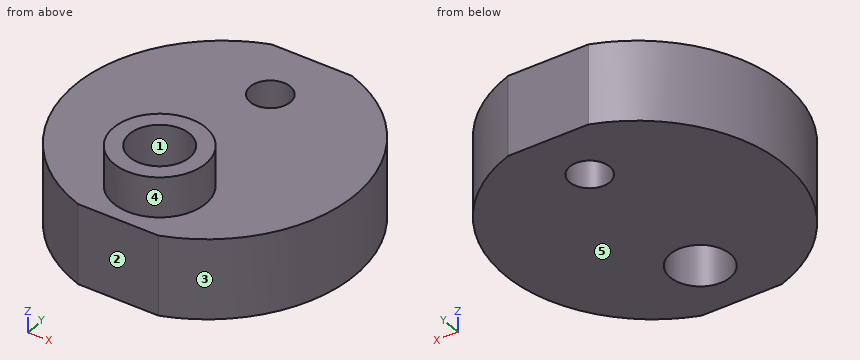
from build123d import *

# Parameters (mm, degrees)
MODEL_R             = 7.3025
MODEL_R_2           = 3.175
MODEL_R_3           = 4.7625
BOSS_EXTRUDE1_DEPTH = 12.7
MODEL_3_R           = 7.3025
MODEL_3_R_2         = 4.7625
BOSS_EXTRUDE2_DEPTH = 19.05


with BuildPart() as part:
    # Model → Boss-Extrude1 (new body)
    # profile 1 of 2: a face of its own
    with BuildSketch(Plane.XY):
        with BuildLine():
            Line((277.621999997, 256.159), (264.921999997, 256.159))
            ThreePointArc((264.921999997, 256.159), (249.046999977, 233.934), (264.921999997, 211.709))
            Line((264.921999997, 211.709), (277.621999997, 211.709))
            ThreePointArc((277.621999997, 211.709), (293.497000017, 233.934), (277.621999997, 256.159))
        make_face()
        with Locations((271.271999997, 221.234)):
            Circle(MODEL_R, mode=Mode.SUBTRACT)
        with Locations((271.271999997, 246.634)):
            Circle(MODEL_R_2, mode=Mode.SUBTRACT)
    # profile 2 of 2: a face of its own
    with BuildSketch(Plane.XY):
        with Locations((271.271999997, 221.234)):
            Circle(MODEL_R)
        with Locations((271.271999997, 221.234)):
            Circle(MODEL_R_3, mode=Mode.SUBTRACT)
    extrude(amount=BOSS_EXTRUDE1_DEPTH)

    # Model_3 → Boss-Extrude2 (add)
    with BuildSketch(Plane.XY):
        with Locations(Location((271.271999997, 221.234, 0), (0, 0, 180))):
            Circle(MODEL_3_R)
        with Locations((271.271999997, 221.234)):
            Circle(MODEL_3_R_2, mode=Mode.SUBTRACT)
    extrude(amount=BOSS_EXTRUDE2_DEPTH)


solid = part.part
For this review, take the finished solid that the model builds, in its own axes (mm). Face numbers are marked on the shaded views. A direction names the side the tool comes from. Round coordinates to 2 decimals unless told otherwise and drop trailing zeros. Write each loop counter-clockwise with the first axis right and the second up, starting at its lowest first coordinate (ties: lowest second). Pieces come first, ordered by that corner, then holes. Notation, with made-up numbers: (11.25, 35) -> (17.25, 35) arc R19 cw to (17.25, 69) -> close; hole circle Ø1 at (24.25, 45.5). An arc over 180 degrees is marked (long way). Put each result on its own line as item: value.
Q1. Consider section B-B on x = 272.5. State the section outline as (y, z) points.
Determined:
outline: (211.71, 0) -> (216.63, 0) -> (216.63, 19.05) -> (214.04, 19.05) -> (214.04, 12.7) -> (211.71, 12.7) -> close; (225.84, 0) -> (243.71, 0) -> (243.71, 12.7) -> (228.43, 12.7) -> (228.43, 19.05) -> (225.84, 19.05) -> close; (249.56, 0) -> (256.16, 0) -> (256.16, 12.7) -> (249.56, 12.7) -> close
Q2. To check wall thickness, follow L1, parallel to Y at x = 271, z = 5; L2, parallel to X at y = 221, z = 17.25; L3, parallel to Z at x = 269, y = 236.5. State the ranges of each line that lie inside material, in increasing order. Write a range as [from, to].
Determined:
L1: y = [211.71, 216.48], [225.99, 243.47], [249.8, 256.16]
L2: x = [263.97, 266.52], [276.03, 278.57]
L3: z = [0, 12.7]
Q3. Consider section C-C on z = 9. Give the number of separate pieces and of enclosed holes in the cut face, and give its area (3 significant figures).
Determined:
separate pieces: 1
enclosed holes: 2
area: 1,490 mm^2
Q4. Machinability: for the marked faces 4 and 5, which of the approach directions +Z, -Z, +X, -X, +Y, -Y give a long, thin tool a straight path to every point of the face, cutting with its end or side? Answer none if there is none.
Determined:
face 4: +Z
face 5: -Z, +X, -X, +Y, -Y
Q5. Clearance check with flat-ended pins moving along their axes: pin 1 Ø6 at (y, z) = (229, 3.5) entering from +X; pin 2 Ø8 at (x, y) = (286, 239) entering from +Z; pin 3 Ø4 at (y, z) = (220, 8) entering from -X. State where each tip first meets the part, or that it passes through.
Determined:
pin 1: stops at x = 293.42
pin 2: stops at z = 12.7
pin 3: stops at x = 252.3
Q6. The part is to be moulded in two halves that separate along X. For the marked faces 1, 2 and 3, say which applies: released by +X, released by -X, zero draft, split by the parting line, or undercut.
Determined:
face 1: undercut
face 2: zero draft
face 3: released by +X
Q7. Consider section A-A on y = 246. State the section outline as (x, z) points, and give its area (3 significant figures).
Determined:
outline: (252.38, 0) -> (268.16, 0) -> (268.16, 12.7) -> (252.38, 12.7) -> close; (274.38, 0) -> (290.16, 0) -> (290.16, 12.7) -> (274.38, 12.7) -> close
area: 401 mm^2
Q8. Consider section D-D on y = 236. State the section outline as (x, z) points, and give its area (3 significant figures).
Determined:
outline: (249.14, 0) -> (293.41, 0) -> (293.41, 12.7) -> (249.14, 12.7) -> close
area: 562 mm^2
